Part model, mm, in its own coordinate system. Face numbers are marked on the shaded views. A direction names the side the tool comes from. Give positions to 0.01 mm unless a question says otherwise; leave off trailing zeros. Write each loop counter-clockwise with the first axis right and the second up, starting at its lowest first coordinate (ties: lowest second). Pieces come first, ordered by that corner, then holes.
from build123d import *

# Parameters (mm, degrees)
SKETCH_1_R               = 6.325
EXTRUDE_1_DEPTH          = 15
SKETCH_2_W               = 28.5
SKETCH_2_H               = 18
EXTRUDE_2_DEPTH          = 3
EXTRUDE_START            = 14.25
SKETCH_4_R               = 1.6
EXTRUDE_3_DEPTH          = 7
EXTRUDE_START_2          = -7.25
SKETCH_4_2_R             = 1.6
EXTRUDE_4_DEPTH          = 7
EXTRUDE_START_3          = -7
EXTRUDE_5_DEPTH          = 7
SKETCH_7_R               = 1.75
CUT_EXTRUDE_1_DEPTH      = 65.242217427
CHAMFER_1_SIZE           = 1
CHAMFER_2_SIZE           = 1
CUT_EXTRUDE_2_DEPTH      = 64.238141181
CUT_EXTRUDE_2_DEPTH_BACK = 64.238141181
SKETCH_8_R               = 1.65
CUT_EXTRUDE_START        = -18
CUT_EXTRUDE_3_OUTLINE_W  = 7
CUT_EXTRUDE_3_OUTLINE_H  = 43
CUT_EXTRUDE_3_OUTLINE_R  = 1.75
CUT_EXTRUDE_3_DEPTH      = 23


# Read off the part's stored shape, not the designer's step: ｶｯﾄ - 押し出し3
with BuildPart() as part:
    # ｽｹｯﾁ1 → ﾎﾞｽ - 押し出し1 (new body)
    with BuildSketch(Plane.XY):
        Circle(SKETCH_1_R)
    extrude(amount=EXTRUDE_1_DEPTH)

    # ｽｹｯﾁ2 → ﾎﾞｽ - 押し出し2 (add)
    with BuildSketch(Plane.XY.offset(15)):
        Rectangle(SKETCH_2_W, SKETCH_2_H)
    extrude(amount=EXTRUDE_2_DEPTH)

    # ｽｹｯﾁ4 → ﾎﾞｽ - 押し出し3 (add)
    with BuildSketch(Plane(origin=(0, 0, 0), x_dir=(0, 0, -1), z_dir=(1, 0, 0)).offset(EXTRUDE_START)):
        with BuildLine():
            Line((-54.074074074, 13.913518208), (-28, 9))
            Line((-28, 9), (-18, 9))
            Line((-18, 9), (-18, -9))
            Line((-18, -9), (-56.624751337, 4.271344473))
            ThreePointArc((-56.624751337, 4.271344473), (-59.833732287, 10.278683768), (-54.074074074, 13.913518208))
        make_face()
        with Locations(Location((-55, 9, 0), (0, 0, 270))):
            Circle(SKETCH_4_R, mode=Mode.SUBTRACT)
    extrude(amount=-EXTRUDE_3_DEPTH)

    # ｽｹｯﾁ4<2> → ﾎﾞｽ - 押し出し4 (add)
    with BuildSketch(Plane(origin=(0, 0, 0), x_dir=(0, 0, -1), z_dir=(1, 0, 0)).offset(EXTRUDE_START_2)):
        with BuildLine():
            Line((-54.074074074, 13.913518208), (-28, 9))
            Line((-28, 9), (-18, 9))
            Line((-18, 9), (-18, -9))
            Line((-18, -9), (-56.624751337, 4.271344473))
            ThreePointArc((-56.624751337, 4.271344473), (-59.833732287, 10.278683768), (-54.074074074, 13.913518208))
        make_face()
        with Locations(Location((-55, 9, 0), (0, 0, 270))):
            Circle(SKETCH_4_2_R, mode=Mode.SUBTRACT)
    extrude(amount=-EXTRUDE_4_DEPTH)

    # ｽｹｯﾁ5 → ﾎﾞｽ - 押し出し5 (add)
    with BuildSketch(Plane.ZY.offset(14.25).offset(EXTRUDE_START_3)):
        with BuildLine():
            Line((18, -9), (33.823085464, -9))
            Line((33.823085464, -9), (57.5, 4.669872981))
            ThreePointArc((57.5, 4.669872981), (57.071979643, 4.44951647), (56.624751337, 4.271344473))
            Line((56.624751337, 4.271344473), (18, -9))
        make_face()
    extrude_5 = extrude(amount=EXTRUDE_5_DEPTH)

    # ﾐﾗｰ1: ﾎﾞｽ - 押し出し5 across plane
    add(extrude_5.mirror(Plane(origin=(0, 0, 0), x_dir=(0, 0, 1), z_dir=(1, 0, 0))))

    # ｽｹｯﾁ7 → ｶｯﾄ - 押し出し1 (cut, through all)
    with BuildSketch(Plane(origin=(0, 9, 0), x_dir=(1, 0, 0), z_dir=(0, 1, 0))):
        with Locations(Location((10.75, -23, 0), (0, 0, 270))):
            Circle(SKETCH_7_R)
        with Locations(Location((-10.75, -23, 0), (0, 0, 90))):
            Circle(SKETCH_7_R)
    extrude(amount=-CUT_EXTRUDE_1_DEPTH, mode=Mode.SUBTRACT)

    # 面取り1
    chamfer_1_edges = [part.edges().sort_by_distance(p)[0] for p in [
        (14.25, 11.456759104, 41.037037037),
        (-14.25, 11.456759104, 41.037037037),
        (-14.25, 10.737621487, 59.688354889),
        (-14.25, -2.165063509, 45.661542732),
        (14.25, 0, 15),
        (14.25, -9, 24.411542732),
        (0, 9, 15),
        (14.25, 10.737621487, 59.688354889),
        (14.25, 9, 21.5),
        (-14.25, 0, 15),
        (14.25, -2.165063509, 45.661542732),
        (-14.25, 9, 21.5),
        (0, -9, 15),
        (-14.25, -9, 24.411542732),
    ]]
    chamfer(chamfer_1_edges, length=CHAMFER_1_SIZE)

    # 面取り2
    chamfer_2_edges = [part.edges().sort_by_distance(p)[0] for p in [
        (-6.325, 0, 0),
    ]]
    chamfer(chamfer_2_edges, length=CHAMFER_2_SIZE)

    # ｽｹｯﾁ8 → ｶｯﾄ - 押し出し2 (cut, two sides: drawn at the far end of the back side and taken through both)
    with BuildSketch(Plane(origin=(0, 0, 0), x_dir=(0, 0, -1), z_dir=(1, 0, 0)).offset(-CUT_EXTRUDE_2_DEPTH_BACK)):
        with Locations(Location((-7.5, 0, 0), (0, 0, 180))):
            Circle(SKETCH_8_R)
    extrude(amount=CUT_EXTRUDE_2_DEPTH + CUT_EXTRUDE_2_DEPTH_BACK, mode=Mode.SUBTRACT)

    # ｶｯﾄ - 押し出し3 outline → ｶｯﾄ - 押し出し3 (cut)
    # profile 1 of 2: a face of its own
    with BuildSketch(Plane(origin=(0, 9, 0), x_dir=(1, 0, 0), z_dir=(0, 1, 0)).offset(CUT_EXTRUDE_START)):
        with Locations((-10.75, -39.5)):
            Rectangle(CUT_EXTRUDE_3_OUTLINE_W, CUT_EXTRUDE_3_OUTLINE_H)
        with Locations((-10.75, -23)):
            Circle(CUT_EXTRUDE_3_OUTLINE_R, mode=Mode.SUBTRACT)
    # profile 2 of 2: a face of its own
    with BuildSketch(Plane(origin=(0, 9, 0), x_dir=(1, 0, 0), z_dir=(0, 1, 0)).offset(CUT_EXTRUDE_START)):
        with Locations((10.75, -39.5)):
            Rectangle(CUT_EXTRUDE_3_OUTLINE_W, CUT_EXTRUDE_3_OUTLINE_H)
        with Locations((10.75, -23)):
            Circle(CUT_EXTRUDE_3_OUTLINE_R, mode=Mode.SUBTRACT)
    extrude(amount=CUT_EXTRUDE_3_DEPTH, mode=Mode.SUBTRACT)


solid = part.part
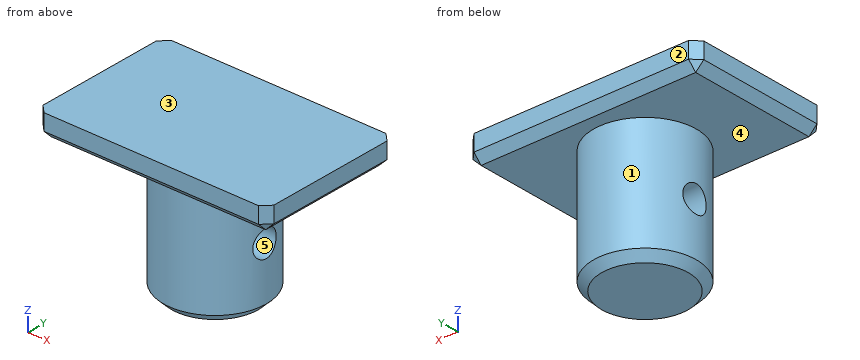
1) 3-axis set-ups, long thin cutter, end or side, ignore diameter. For the marked faces 1 and 2: which of +Z, -Z, +X, -X, +Y, -Y reach the whole face in a straight line?
Check result:
face 1: -Z
face 2: +Z, -Z, +X, -X, +Y
2) Mould opens along Z. For the marked faces 3, 4 and 5 say: +Z half, -Z half, draft (parallel to the pull), parting line (faces both ways), or undercut.
Check result:
face 3: +Z half
face 4: -Z half
face 5: undercut
3) Flat gauge pins, fed straight in: P1, Ø8, axis at x = -3.5, z = 2.5, coming from the -Y side (3 decimals); P2, Ø8, axis at y = -3.5, z = 8.5, coming from the +X side (3 decimals); P3, Ø5, axis at x = 6.5, z = 3, coming from the +Y side. Where does each tip first touch, or does it go through?
Check result:
P1: stops at y = -6.325
P2: stops at x = 6.325
P3: stops at y = 4.9
4) Saw through at A-A (y = 0). Write the cut outline in (x, z) (3 decimals).
Check result:
outline: (-14.25, 16) - (-13.25, 15) - (-6.325, 15) - (-6.325, 9.15) - (6.325, 9.15) - (6.325, 15) - (13.25, 15) - (14.25, 16) - (14.25, 18) - (-14.25, 18) - close; (-6.325, 1) - (-5.325, 0) - (5.325, 0) - (6.325, 1) - (6.325, 5.85) - (-6.325, 5.85) - close
5) Saw through at C-C (x = -9.75). Write the cut outline in (y, z).
Check result:
outline: (-9, 16) - (-8, 15) - (8, 15) - (9, 16) - (9, 18) - (-9, 18) - close
6) Saw through at B-B (x = 0). Write the cut outline in (y, z) (3 decimals), and give its area (3 significant figures).
Check result:
outline: (-9, 16) - (-8, 15) - (-6.325, 15) - (-6.325, 1) - (-5.325, 0) - (5.325, 0) - (6.325, 1) - (6.325, 15) - (8, 15) - (9, 16) - (9, 18) - (-9, 18) - close; hole circle Ø3.3 at (0, 7.5)
area: 233 mm2
7) Saw through at D-D (y = -7). Write the cut outline in (x, z).
Check result:
outline: (-14.25, 16) - (-13.25, 15) - (13.25, 15) - (14.25, 16) - (14.25, 18) - (-14.25, 18) - close
8) Drill centre lines: L1, parallel to Z at x = -9.5, y = -6.5; L2, parallel to Y at x = 2.75, z = 7.5; L3, parallel to Y at x = -2, z = 7.5. Where is each one in solid material? Low to high.
Check result:
L1: z = 15 to 18
L2: y = -5.7 to -1.65, 1.65 to 5.7
L3: y = -6 to -1.65, 1.65 to 6
